Here's the drawing with two shaded views (mm, measured from the low corner). I have some questions. Coordinates: 2 decimals unless noted, no trailing zeros. Loops run counter-clockwise (first coordinate to the right, second up) from the corner with the lowest first, then second, coordinate; pieces in that order, holes last. Notation, with made-up numbers: (-11.5, 10.5) - (46.5, 10.5) arc R14 ccw to (46.5, 14.5) - close; hole circle Ø9 at (21, 1). An arc over 180 degrees is marked (long way). One line per item, written item: value. Start each with the question number.
(1) I'm going to push flat-ended pins straight in: P1, Ø1.6, axis at x = 81, y = 2, coming from the +Z side (1 decimal); P2, Ø1, axis at x = 87.5, y = 1, coming from the +Z side; P3, Ø1.5, axis at y = 2.5, z = 15, coming from the -X side. Where does each tip first touch, or does it pass through?
(2) If I drill on line 1 along X through (y, z) = (2.5, 6.75); line 2 along Z through (x, y) = (74.5, 0.55) (1 decimal), over which ranges is the centre line in solid material (lowest first)? Write a range as from..to.
(3) If we section it at A-A on x = 82.5: Write out the boundary of the cut face in (y, z) (1 decimal).
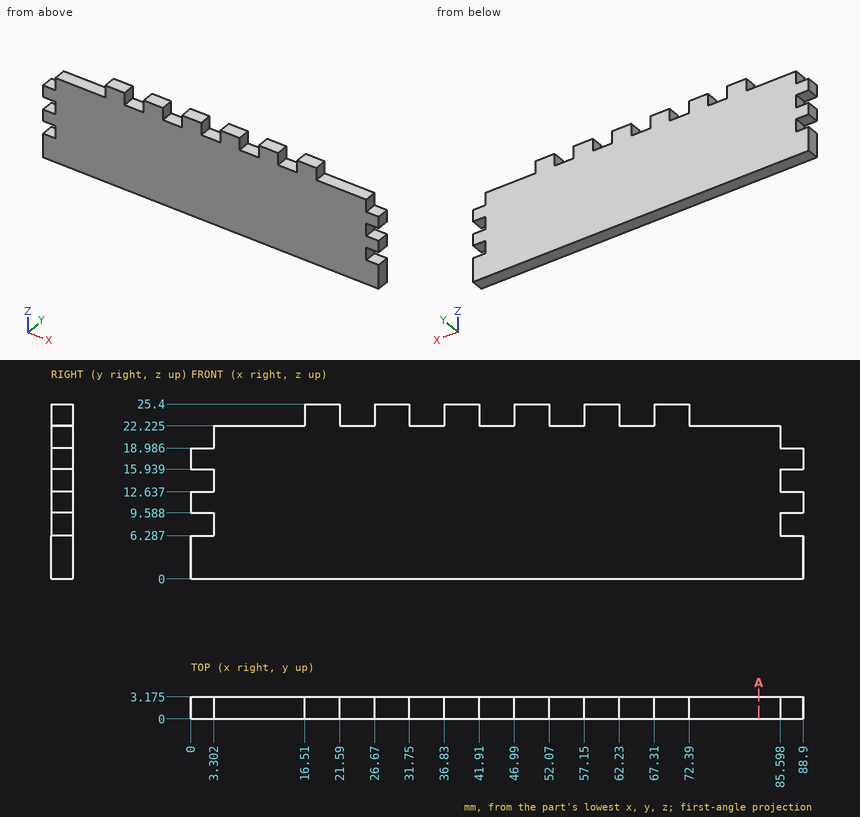
Values:
1. P1: stops at z = 22.2
1. P2: stops at z = 18.99
1. P3: stops at x = 3.3
2. line 1: x = 3.3..85.6
2. line 2: z = 0..22.2
3. outline: (0, 0) - (3.2, 0) - (3.2, 22.2) - (0, 22.2) - close
